Input: dimensioned drawing with shaded views. Units: mm. Origin: part minimum x, y, z. A direction names the side the tool comes from. Round coordinates to 2 decimals unless told otherwise and drop trailing zeros. Write each loop counter-clockwise with the first axis right and the second up, starting at its lowest first coordinate (ties: lowest second). Pieces come first, ordered by that corner, then holes. Notation, with made-up numbers: M 73,77.25 L 127,77.25 A18 ccw 127,85.25 Z; hole C -40,59 d7. An arc over 180 degrees is marked long. Answer as CSV lines item,"result". Start each with the question number.
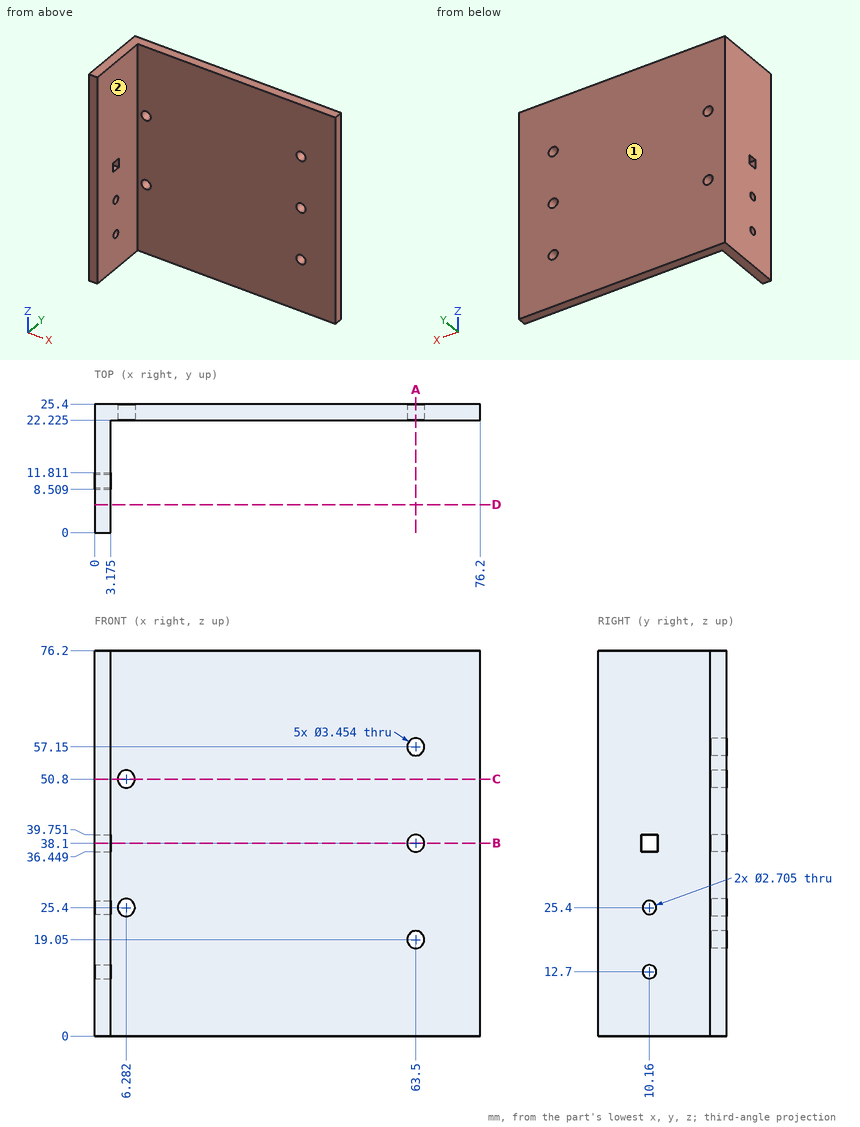
Item 1: Cut plane D-D, the plane y = 5.5. Return loops of the section in (x, z) (1 decimal), plus the area to 3 significant figures.
Item 2: Cut plane C-C, the plane z = 50.8. Return loops of the section in (x, y) (1 decimal).
Item 3: Cut plane A-A, the plane x = 63.5. Return loops of the section in (y, z) (1 decimal), plus the area to 3 significant figures.
Item 4: Access query for the marked faces 1 and 2. Directions: +Z, -Z, +X, -X, +Y, -Y. A direction counts if a zero-diameter tool reaches every point of the face in a straight line with its end or side. Return the directions, or none.
Item 5: Cut plane B-B, the plane z = 38.1. Return loops of the section in (x, y) (1 decimal).
Item 6: Line query: line 1 (Z direction, x = 63.5, y = 23.3); line 2 (Y direction, x = 1.5, z = 25.4); line 3 (X direction, y = 24, z = 50.8) (1 decimal). Output: solid intervals per line, ascending. Write a range as [from, to].
Item 7: Pin query (flat end, axial travel): pin 1 Ø6.5 at (y, z) = (14, 47.5) entering from +X (3 decimals); pin 2 Ø4 at (x, z) = (6.28, 50.8) entering from -Y (3 decimals). Return the tip coordinate at first contact, or that it passes through.
Results list:
1,outline,"M 0,0 L 3.2,0 L 3.2,76.2 L 0,76.2 Z"
1,area,"242 mm²"
2,outline,"M 0,0 L 3.2,0 L 3.2,22.2 L 4.6,22.2 L 4.6,25.4 L 0,25.4 Z; M 8,22.2 L 76.2,22.2 L 76.2,25.4 L 8,25.4 Z"
3,outline,"M 22.2,0 L 25.4,0 L 25.4,17.3 L 22.2,17.3 Z; M 22.2,20.8 L 25.4,20.8 L 25.4,36.4 L 22.2,36.4 Z; M 22.2,39.8 L 25.4,39.8 L 25.4,55.4 L 22.2,55.4 Z; M 22.2,58.9 L 25.4,58.9 L 25.4,76.2 L 22.2,76.2 Z"
3,area,"209 mm²"
4,face 1,"+Z, -Z, +X, -X, +Y"
4,face 2,"+Z, -Z, +X, -Y"
5,outline,"M 0,0 L 3.2,0 L 3.2,8.5 L 0,8.5 Z; M 0,11.8 L 3.2,11.8 L 3.2,22.2 L 61.8,22.2 L 61.8,25.4 L 0,25.4 Z; M 65.2,22.2 L 76.2,22.2 L 76.2,25.4 L 65.2,25.4 Z"
6,line 1,"[0, 17.32], [20.78, 36.37], [39.83, 55.42], [58.88, 76.2]"
6,line 2,"[0, 8.81], [11.51, 25.4]"
6,line 3,"[0, 4.6], [8, 76.2]"
7,pin 1,"x = 3.175"
7,pin 2,"y = 22.225"
